```python
from build123d import *

# Parameters (mm, degrees)
PAD_DEPTH    = 11
CHAMFER_SIZE = 3
FILLET_R     = 2


with BuildPart() as part:
    # Sketch → Pad (new body)
    with BuildSketch(Plane.XY):
        Polygon((-22.735205, -3.599016), (-22.735205, -8.599016), (10.264795, -8.599016), (10.264795, 18.400984), (15.464795, 18.400984), (15.464795, -8.599016), (18.464795, -8.599016), (18.464795, 21.400984), (7.264795, 21.400984), (7.264795, -3.599016), align=None)
    extrude(amount=PAD_DEPTH)

    # Chamfer
    chamfer_edges = [part.edges().sort_by_distance(p)[0] for p in [
        (-6.235205, -8.599016, 0),
        (-6.235205, -8.599016, 11),
    ]]
    chamfer(chamfer_edges, length=CHAMFER_SIZE)

    # Fillet
    fillet_edges = [part.edges().sort_by_distance(p)[0] for p in [
        (18.464795, 21.400984, 5.5),
        (7.264795, 21.400984, 5.5),
    ]]
    fillet(fillet_edges, radius=FILLET_R)


solid = part.part
```
Geometry check sheet. Reference: the model listing, model coordinates, mm. A direction names the side the tool comes from. Coordinates: 2 decimals unless noted, no trailing zeros. Order: outer loops, then holes, each group sorted by start corner. A loop starts at its lowest first (then second) coordinate and runs counter-clockwise, first axis right, second up. Notation, with made-up numbers: M 0,-24 L 33,-24 A23 cw 33,-9 Z; hole C -35,27 d11. An arc over 180 degrees is marked long. Answer as a JSON object with one key per item and string values.
Q1. Cross-section at D-D on z = 7.25. Record the cut outline in (x, y).
Results are:
{"outline": "M -22.74,-8.6 L 10.26,-8.6 L 10.26,18.4 L 15.46,18.4 L 15.46,-8.6 L 18.46,-8.6 L 18.46,19.4 A2 ccw 16.46,21.4 L 9.26,21.4 A2 ccw 7.26,19.4 L 7.26,-3.6 L -22.74,-3.6 Z"}
Q2. Release check for a two-part mould opening along X. For faces 1 (the flat face through (-6.5, -7.1, 1.5)), 2 (the flat face through (10.265, 5, 5)), 3 (the flat face through (7.265, 8, 5)) record: released by +X, released by -X, zero draft, split by the parting line, or undercut.
Results are:
{"face 1": "zero draft", "face 2": "undercut", "face 3": "released by -X"}
Q3. Depth check by flat-ended pin: pin 1 Ø5.5 at (y, z) = (3.5, 8) entering from -X; pin 2 Ø4 at (x, z) = (14, 4) entering from -Y. Enter the tip coordinate at first touch or a pass-through.
Results are:
{"pin 1": "stops at x = 7.26", "pin 2": "stops at y = -8.6"}
Q4. Scan lines: line 1 (X direction, y = 2, z = 3); line 2 (X direction, y = -6.5, z = 3.5); line 3 (Y direction, x = -12.5, z = 7). Record each from-to range of solid material in increasing order.
Results are:
{"line 1": "x = 7.26 to 10.26, 15.46 to 18.46", "line 2": "x = -22.74 to 10.26, 15.46 to 18.46", "line 3": "y = -8.6 to -3.6"}
Q5. Cross-section at A-A on y = -5. Record the cut outline in (x, z), and give its area (3 significant figures).
Results are:
{"outline": "M -22.74,0 L 10.26,0 L 10.26,11 L -22.74,11 Z; M 15.46,0 L 18.46,0 L 18.46,11 L 15.46,11 Z", "area": "396 mm²"}
Q6. Tool access check on faces 4 (the flat face through (-6.5, -7.1, 9.5)), 5 (the flat face through (13, 18.401, 5)), 6 (the flat face through (10, 6, 0)), 7 (the flat face through (-8, -3.599, 5)). Record the directions out of +Z, -Z, +X, -X, +Y, -Y that give a thin tool (end or side, any length) a straight path to the whole face; none if there is none.
Results are:
{"face 4": "+Z, -X, -Y", "face 5": "+Z, -Z, -Y", "face 6": "-Z, +X, -X, +Y, -Y", "face 7": "+Z, -Z, -X, +Y"}
Q7. Cross-section at C-C on x = -14. Record the cut outline in (y, z).
Results are:
{"outline": "M -8.6,3 L -5.6,0 L -3.6,0 L -3.6,11 L -5.6,11 L -8.6,8 Z"}
Q8. Cross-section at B-B on y = 0. Record the cut outline in (x, z).
Results are:
{"outline": "M 7.26,0 L 10.26,0 L 10.26,11 L 7.26,11 Z; M 15.46,0 L 18.46,0 L 18.46,11 L 15.46,11 Z"}
